Read the model definition and answer for the solid it produces. Units are mm, in the model's axes. A direction names the side the tool comes from. Give positions to 0.01 mm unless a question says otherwise; leave off trailing zeros. Order: outer loops, then holes, each group sorted by start corner. A loop starts at its lowest first (then second) coordinate and runs counter-clockwise, first axis right, second up. Notation, with made-up numbers: (-13.75, 4.5) - (20.25, 4.5) arc R30 cw to (20.25, 40.5) - close; hole circle Ø2 at (82, 29.5). An arc over 180 degrees is marked (long way). Write each question's results on one line, items separated by ' | '.
from build123d import *

# Parameters (mm, degrees)
F1_DEPTH       = 76.2
F3_D           = 4.9784
F3_CSINK_D     = 9.1186
F3_CSINK_ANGLE = 82
F5_D           = 5.6134
F5_CSINK_D     = 10.4394
F5_CSINK_ANGLE = 82
F6_W           = 38.1
F6_H           = 79.375
F7_DEPTH       = 50.801


with BuildPart() as f1:
    # F0 (on Front) → F1 (new body)
    with BuildSketch(Plane.XZ):
        Polygon((-50.8, 0), (0, 0), (0, 101.6), (-6.35, 101.6), (-6.35, 6.35), (-50.8, 6.35), align=None)
    extrude(amount=-F1_DEPTH)

    # F3 (through all)
    with Locations(Plane(origin=(-6.35, 0, 0), x_dir=(0, -1, 0), z_dir=(-1, 0, 0))):
        with Locations((-9.525, 92.075), (-28.575, 34.925)):
            CounterSinkHole(F3_D / 2, F3_CSINK_D / 2, counter_sink_angle=F3_CSINK_ANGLE)

    # F5 (through all)
    with Locations(Plane.XY.offset(6.35)):
        with Locations((-25.4, 25.4), (-27.0796256672, 50.8)):
            CounterSinkHole(F5_D / 2, F5_CSINK_D / 2, counter_sink_angle=F5_CSINK_ANGLE)

    # F6 (on face) → F7 (cut, through all)
    with BuildSketch(Plane.YZ):
        with Locations((57.15, 61.9125)):
            Rectangle(F6_W, F6_H)
    extrude(amount=-F7_DEPTH, mode=Mode.SUBTRACT)


solid = f1.part
(1) For faces 1 (the face through (-3, 38.1, 61)), 2 (the face through (-4.084, 8.964, 89.547)), 3 (the face through (-6.35, 21, 55)), determine the directions among +Z, -Z, +X, -X, +Y, -Y from which every point of the face is accessible in a straight line to the end or side of a thin tool.
Conclusion:
face 1: +Z, +X, -X, +Y | face 2: -X | face 3: +Z, -X, +Y, -Y
(2) Section C-C (z = 9) is taken. Give the vertices of the cut face in (x, y), plus the area to 3 significant figures.
Conclusion:
outline: (-6.35, 0) - (0, 0) - (0, 76.2) - (-6.35, 76.2) - close | area: 484 mm^2
(3) Section B-B (y = 40) is taken. Give the vertices of the cut face in (x, z) (3 decimals).
Conclusion:
outline: (-50.8, 0) - (0, 0) - (0, 22.225) - (-6.35, 22.225) - (-6.35, 6.35) - (-50.8, 6.35) - close
(4) The mould has two halves that part along Y. Classify faces 4 (the face through (-20, 76.2, 6)), 5 (the face through (-3, 57, 22.225)), 6 (the face through (-4.1, 28.2, 37.5)): pulls with the +Y half, pulls with the -Y half, needs draft (parallel to the pull), parting line crosses it, or undercut.
Conclusion:
face 4: pulls with the +Y half | face 5: needs draft | face 6: undercut
(5) Each of these flat-tipped pins is pushed along its axis until it touches: pin 1 (12 mm diameter, centred on x = -14, z = 76.5, fed in from -Y); pin 2 (5 mm diameter, centred on x = -4, z = 54, fed in from +Y); pin 3 (3 mm diameter, centred on y = 13.5, z = 87, fed in from +X); pin 4 (23 mm diameter, centred on y = 49, z = 54.5, fed in from -X). Where does it stop, or does it pass through?
Conclusion:
pin 1: through | pin 2: y = 38.1 | pin 3: x = 0 | pin 4: x = -6.35
(6) Section D-D (x = -25.4) is taken. State how many separate pieces and enclosed holes the cut face has, plus the area to 3 significant figures.
Conclusion:
separate pieces: 3 | enclosed holes: 0 | area: 405 mm^2
(7) Section A-A (y = 50.8) is taken. Give the vertices of the cut face in (x, z) (3 decimals), plus the area to 3 significant figures.
Conclusion:
outline: (-50.8, 0) - (-29.886, 0) - (-29.886, 3.574) - (-32.299, 6.35) - (-50.8, 6.35) - close; (-24.273, 0) - (0, 0) - (0, 22.225) - (-6.35, 22.225) - (-6.35, 6.35) - (-21.86, 6.35) - (-24.273, 3.574) - close | area: 381 mm^2
(8) Consider probe 1 along X at (y, z) = (25.4, 2.1); probe 2 along Z at (x, y) = (-13, 8); probe 3 along X at (y, z) = (50.8, 2.7). Determine where each line is inside the solid, lowest interval first. Write a range as [from, to].
Conclusion:
probe 1: [-50.8, -28.21], [-22.59, 0] | probe 2: [0, 6.35] | probe 3: [-50.8, -29.89], [-24.27, 0]
